Design review of the part shown in the three views and the two pictorial views. Dimensions are in mm from the part's minimum x, y and z. Give positions to 0.01 mm unless a question says otherwise; leave off trailing zeros. Loops run counter-clockwise (first coordinate to the right, second up) from the corner with the lowest first, then second, coordinate; pieces in that order, holes last. Notation, with made-up numbers: (-38, -23) - (-30, -23) arc R35 ccw to (-30, 12) - close; hole circle Ø4 at (65.25, -34.75). An arc over 180 degrees is marked (long way). Return JSON: item names as keys, results as strings. Group by question number.
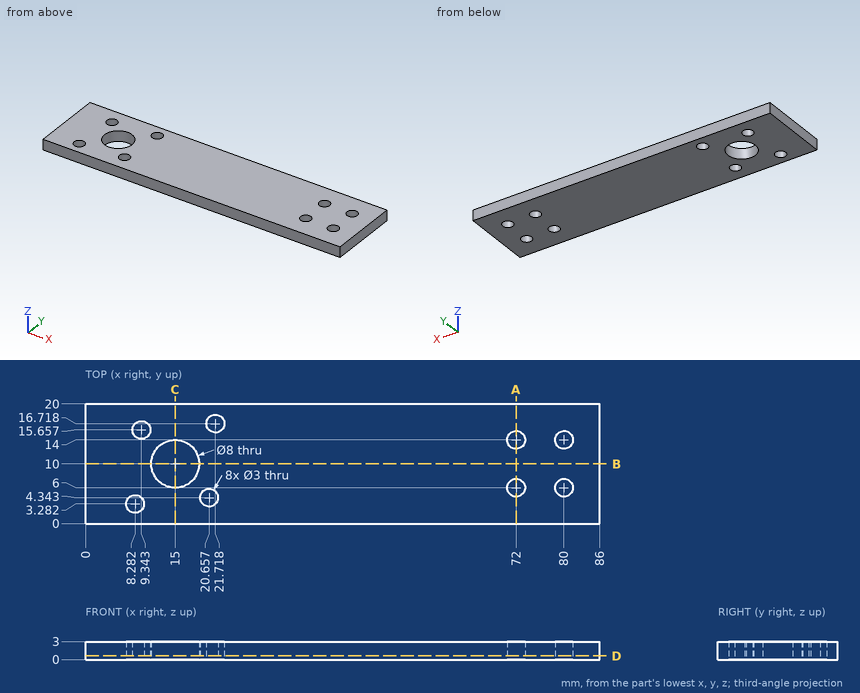
Item 1: Take a section at A-A (x = 72). State the section outline as (y, z) points.
Item 2: Take a section at D-D (z = 0.6). State how many separate pieces and enclosed holes the cut face has, then the cut area to 3 significant figures.
Item 3: For L1, parallel to Y at x = 80, z = 0.8; L2, parallel to X at y = 7, z = 2.55 (1 decimal); L3, parallel to X at y = 15, z = 2.4 (1 decimal), list the stretches that pass through material, from the lowest coordinate up. Write a range as from..to.
Item 4: Take a section at C-C (x = 15). State the section outline as (y, z) points.
Item 5: For P1, Ø2.5, axis at x = 9.34, y = 15.66, coming from the -Z side, flat-tipped, find the tip position at first contact; note if it passes through.
Item 6: Take a section at B-B (y = 10). State the section outline as (x, z) points.
Check sheet entries:
{
 "1": {"outline": "(0, 0) - (4.5, 0) - (4.5, 3) - (0, 3) - close; (7.5, 0) - (12.5, 0) - (12.5, 3) - (7.5, 3) - close; (15.5, 0) - (20, 0) - (20, 3) - (15.5, 3) - close"},
 "2": {"separate pieces": "1", "enclosed holes": "9", "area": "1,610 mm^2"},
 "3": {"L1": "y = 0..4.5, 7.5..12.5, 15.5..20", "L2": "x = 0..12.4, 17.6..70.9, 73.1..78.9, 81.1..86", "L3": "x = 0..8, 10.7..70.9, 73.1..78.9, 81.1..86"},
 "4": {"outline": "(0, 0) - (6, 0) - (6, 3) - (0, 3) - close; (14, 0) - (20, 0) - (20, 3) - (14, 3) - close"},
 "5": {"P1": "passes through"},
 "6": {"outline": "(0, 0) - (11, 0) - (11, 3) - (0, 3) - close; (19, 0) - (86, 0) - (86, 3) - (19, 3) - close"}
}
